The model under review builds one solid part; all positions refer to its coordinate system, in mm. Face numbers are marked on the shaded views. A direction names the side the tool comes from. Coordinates: 2 decimals unless noted, no trailing zeros. Order: outer loops, then holes, each group sorted by start corner. A loop starts at its lowest first (then second) coordinate and runs counter-clockwise, first axis right, second up.
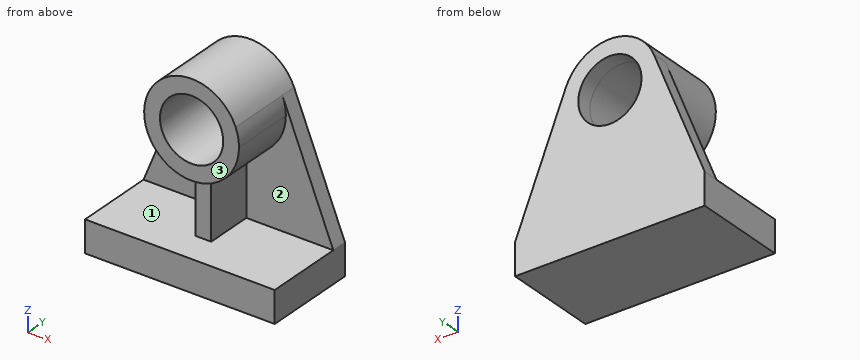
```python
from build123d import *

# Parameters (mm, degrees)
F1_DEPTH      = 25.4
F2_W          = 304.8
F2_H          = 50.8
F3_DEPTH      = 127
F5_R          = 50.8
F6_DEPTH      = 25.401
F7_DEPTH      = 101.6
F8_DEPTH      = 127.001
F8_DEPTH_BACK = 25.401
F10_DEPTH     = 76.2


with BuildPart() as f1:
    # F0 (on Front) → F1 (new body)
    with BuildSketch(Plane.XZ):
        with BuildLine():
            Line((0, 50.8), (0, 0))
            Line((0, 0), (304.8, 0))
            Line((304.8, 0), (304.8, 50.8))
            Line((304.8, 50.8), (223.0993426351, 254))
            ThreePointArc((223.0993426351, 254), (152.4, 301.7739036981), (81.7006573649, 254))
            Line((81.7006573649, 254), (0, 50.8))
        make_face()
    extrude(amount=F1_DEPTH)

    # F2 (on face) → F3 (join)
    with BuildSketch(Plane.XZ.offset(25.4)):
        with Locations((152.4, 25.4)):
            Rectangle(F2_W, F2_H)
    extrude(amount=F3_DEPTH)

    # F5 (on face) → F6 (cut, through all)
    with BuildSketch(Plane.XZ.offset(25.4)):
        with Locations((152.4, 225.5739036981)):
            Circle(F5_R)
    extrude(amount=-F6_DEPTH, mode=Mode.SUBTRACT)

    # F4 (on face) → F7 (join)
    with BuildSketch(Plane.XZ.offset(25.4)):
        with BuildLine():
            ThreePointArc((81.7006573649, 254), (137.9232929986, 150.7617057996), (228.6, 225.5739036981))
            ThreePointArc((228.6, 225.5739036981), (227.2121978984, 240.0506106994), (223.0993426351, 254))
            ThreePointArc((223.0993426351, 254), (152.4, 301.7739036981), (81.7006573649, 254))
        make_face()
    extrude(amount=F7_DEPTH)

    # F5 (on face) → F8 (cut, two sides)
    with BuildSketch(Plane.XZ.offset(25.4)) as f8_sk:
        with Locations((152.4, 225.5739036981)):
            Circle(F5_R)
    extrude(amount=F8_DEPTH, mode=Mode.SUBTRACT)
    extrude(f8_sk.sketch, amount=-F8_DEPTH_BACK, mode=Mode.SUBTRACT)

    # F9 (on face) → F10 (join)
    with BuildSketch(Plane.XZ.offset(25.4)):
        with BuildLine():
            Line((139.7, 150.4396904527), (139.7, 50.8))
            Line((139.7, 50.8), (165.1, 50.8))
            Line((165.1, 50.8), (165.1, 150.4396904527))
            ThreePointArc((165.1, 150.4396904527), (152.4, 149.3739036981), (139.7, 150.4396904527))
        make_face()
    extrude(amount=F10_DEPTH)


solid = f1.part
```
(1) For pin 1 Ø8 at (y, z) = (-77, 231.5) entering from -X; pin 2 Ø20.5 at (x, z) = (153, 118.5) entering from -Y; pin 3 Ø4 at (x, y) = (76.5, -24.5) entering from +Z; pin 4 Ø10 at (y, z) = (-134, 162) entering from -X, all flat-tipped, find the tip position at first contact; note any pin that passes through.
A:
pin 1: stops at x = 76.22
pin 2: stops at y = -101.6
pin 3: stops at z = 246.04
pin 4: passes through
(2) Wall thickness on probe 1 along Z at (x, y) = (152.4, -11); probe 2 along Z at (x, y) = (185, -65); probe 3 along Z at (x, y) = (198, -51): over which ranges is each line inside the solid? List them lowest first.
A:
probe 1: z = 0 to 174.77, 276.37 to 301.77
probe 2: z = 0 to 50.8, 156.7 to 186.61, 264.53 to 294.45
probe 3: z = 0 to 50.8, 164.52 to 203.18, 247.96 to 286.62
(3) We need section C-C, the plane z = 212. Write out the cut boundary in (x, y).
A:
outline: (64.81, -25.4) - (77.42, -25.4) - (77.42, -127) - (103.45, -127) - (103.45, 0) - (64.81, 0) - close; (201.35, -127) - (227.38, -127) - (227.38, -25.4) - (239.99, -25.4) - (239.99, 0) - (201.35, 0) - close
(4) We need section A-A, the plane y = -107. Write out the cut boundary in (x, z).
A:
outline: (0, 0) - (304.8, 0) - (304.8, 50.8) - (0, 50.8) - close; circle Ø152.4 at (152.4, 225.57); hole circle Ø101.6 at (152.4, 225.57)
(5) We need section D-D, the plane y = -41. Write out the cut boundary in (x, z), and give its area (3 significant figures).
A:
outline: (0, 0) - (304.8, 0) - (304.8, 50.8) - (165.1, 50.8) - (165.1, 150.44) arc R76.2 ccw (long way) to (139.7, 150.44) - (139.7, 50.8) - (0, 50.8) - close; hole circle Ø101.6 at (152.4, 225.57)
area: 28,100 mm2
(6) We need section B-B, the plane x = 152.4. Write out the cut boundary in (y, z), and give its area (3 significant figures).
A:
outline: (-152.4, 0) - (0, 0) - (0, 174.77) - (-127, 174.77) - (-127, 149.37) - (-101.6, 149.37) - (-101.6, 50.8) - (-152.4, 50.8) - close; (-127, 276.37) - (0, 276.37) - (0, 301.77) - (-127, 301.77) - close
area: 24,200 mm2
(7) Machinability: for the marked faces 1, 2 and 3, which of the approach directions +Z, -Z, +X, -X, +Y, -Y give a long, thin tool a straight path to every point of the face, cutting with its end or side? Answer none if there is none.
A:
face 1: -Y
face 2: +X, -Y
face 3: +Z, +X, -X, -Y
